from build123d import *

# Parameters (mm, degrees)
F0_W     = 25.4
F0_H     = 25.4
F1_DEPTH = 50.8
F2_R     = 10.16
F3_DEPTH = 50.801


with BuildPart() as f1:
    # F0 (on Front) → F1 (new body)
    with BuildSketch(Plane.XZ):
        with Locations((0.829598, -0.711867)):
            Rectangle(F0_W, F0_H)
    extrude(amount=F1_DEPTH)

    # F2 (on face) → F3 (cut, through all)
    with BuildSketch(Plane.XZ.offset(50.8)):
        Circle(F2_R)
    extrude(amount=-F3_DEPTH, mode=Mode.SUBTRACT)


solid = f1.part
Verification items for the finished model (mm, model axes). Coordinates: 2 decimals unless noted, no trailing zeros. Write each loop counter-clockwise with the first axis right and the second up, starting at its lowest first coordinate (ties: lowest second). Pieces come first, ordered by that corner, then holes. Notation, with made-up numbers: (30, 74.25) - (76, 74.25) arc R15 cw to (76, 87.25) - close; hole circle Ø2 at (14, 4.5). An arc over 180 degrees is marked (long way). Answer as a JSON object with one key per item and string values.
(1) Cross-section at A-A on z = 0. Record the cut outline in (x, y).
Report:
{"outline": "(-11.87, -50.8) - (-10.16, -50.8) - (-10.16, 0) - (-11.87, 0) - close; (10.16, -50.8) - (13.53, -50.8) - (13.53, 0) - (10.16, 0) - close"}
(2) Cross-section at B-B on x = 0. Record the cut outline in (y, z), plus the area to 3 significant figures.
Report:
{"outline": "(-50.8, -13.41) - (0, -13.41) - (0, -10.16) - (-50.8, -10.16) - close; (-50.8, 10.16) - (0, 10.16) - (0, 11.99) - (-50.8, 11.99) - close", "area": "258 mm^2"}
(3) Gauge pin test, flat end, axial feed: pin 1 Ø6 at (x, z) = (5, 0.5) entering from -Y. Record the tip position at first contact, or that the pin passes through.
Report:
{"pin 1": "through"}
(4) Thickness scan on line 1 along Z through (x, y) = (0, -31.5); line 2 along Z through (x, y) = (0.5, -33); line 3 along X through (y, z) = (-20, 2.5). Record the ranges inside material, lowest first.
Report:
{"line 1": "-13.41 to -10.16, 10.16 to 11.99", "line 2": "-13.41 to -10.15, 10.15 to 11.99", "line 3": "-11.87 to -9.85, 9.85 to 13.53"}
(5) Cross-section at C-C on y = -11.5. Record the cut outline in (x, z).
Report:
{"outline": "(-11.87, -13.41) - (13.53, -13.41) - (13.53, 11.99) - (-11.87, 11.99) - close; hole circle Ø20.32 at (0, 0)"}
(6) Mould release check, pull along Z, two halves, no side actions. Record for faces 1 (the cylindrical face through (-1.323, -25.756, 10.074)), 2 (the flat face through (1, -25, -13.412)), 3 (the flat face through (6, 0, -9)): pulls with the +Z half, pulls with the -Z half, needs draft (parallel to the pull), parting line crosses it, or undercut.
Report:
{"face 1": "undercut", "face 2": "pulls with the -Z half", "face 3": "needs draft"}
